Could you check a few things on this model? Use its own coordinates, in mm. Face numbers are marked on the shaded views. A direction names the side the tool comes from. Coordinates: 2 decimals unless noted, no trailing zeros. Write each loop counter-clockwise with the first axis right and the second up, starting at its lowest first coordinate (ties: lowest second). Pieces come first, ordered by that corner, then holes. Notation, with made-up numbers: M 5.5,26.25 L 29.5,26.25 A22 ccw 29.5,49.25 Z; hole C 58,89.25 d7. An arc over 180 degrees is marked long. Answer as CSV lines item,"result". Start each with the question number.
Item 1: We'd pull the mould along Z, two halves only. Please class the marked faces 3, 4, 5 and 6: +Z half, -Z half, draft (parallel to the pull), parting line (faces both ways), or undercut.
Item 2: On a 3-axis mill with a long thin cutter (end or side, diameter ignored), from which of +Z, -Z, +X, -X, +Y, -Y can I reach the whole of each face in a straight line? I mean the marked faces 1 and 2. Say none if no direction works.
Item 3: Suppose I cut it at B-B, the plane x = 6.5. Write out the boundary of the cut face in (y, z).
Item 4: If I drill on line 1 along X through (y, z) = (-12, 13.5); line 2 along Z through (x, y) = (15, -5.5); line 3 along Y through (x, z) = (1, 33), over which ranges is the centre line in solid material (lowest first)? Write a range as [from, to].
Item 5: I'm going to push a flat-ended pin straight in: P1, Ø10, axis at x = 25.5, z = -10, coming from the -Y side. Where does the tip first touch, or does it pass through?
Item 6: Suppose I cut it at C-C, the plane z = -44.5. Write out the boundary of the cut face in (x, y).
Item 7: Suppose I cut it at A-A, the plane y = -15.25. Write out the boundary of the cut face in (x, z), and give its area (3 significant figures).
```python
from build123d import *

# Parameters (mm, degrees)
F0_W     = 69.494404
F0_H     = 106.984802
F1_DEPTH = 25.4
F2_R     = 5.08
F3_T     = -2.54


with BuildPart() as f1:
    # F0 (on Front) → F1 (new body)
    with BuildSketch(Plane.XZ):
        Rectangle(F0_W, F0_H)
    extrude(amount=F1_DEPTH)

    # F2
    f2_edges = [f1.edges().sort_by_distance(p)[0] for p in [
        (-34.747202, -12.7, 53.492401),
        (-34.747202, -12.7, -53.492401),
        (34.747202, -12.7, 53.492401),
        (34.747202, -12.7, -53.492401),
    ]]
    fillet(f2_edges, radius=F2_R)

    # F3
    f3_openings = [f1.faces().sort_by_distance(p)[0] for p in [
        (0, -25.4, 0),
    ]]
    offset(amount=F3_T, openings=f3_openings)


solid = f1.part
```
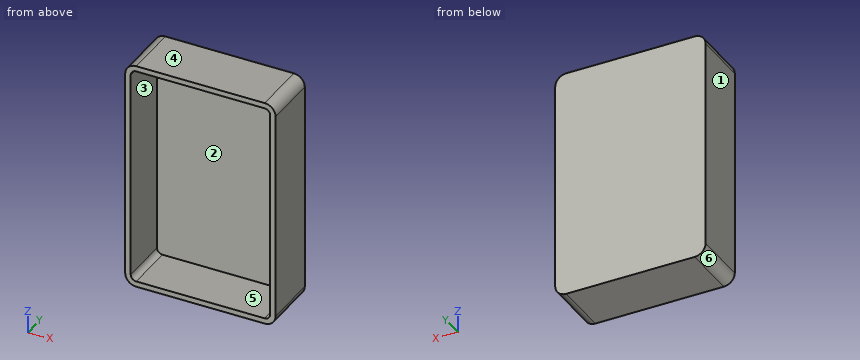
Ans:
1,face 3,"undercut"
1,face 4,"+Z half"
1,face 5,"undercut"
1,face 6,"-Z half"
2,face 1,"+Z, -Z, -X, +Y, -Y"
2,face 2,"-Y"
3,outline,"M -25.4,-53.49 L 0,-53.49 L 0,53.49 L -25.4,53.49 L -25.4,50.95 L -2.54,50.95 L -2.54,-50.95 L -25.4,-50.95 Z"
4,line 1,"x = [-34.75, -32.21], [32.21, 34.75]"
4,line 2,"z = [-53.49, -50.95], [50.95, 53.49]"
4,line 3,"y = [-2.54, 0]"
5,P1,"stops at y = -2.54"
6,outline,"M -34.75,-25.4 L -32.21,-25.4 L -32.21,-2.54 L 32.21,-2.54 L 32.21,-25.4 L 34.75,-25.4 L 34.75,0 L -34.75,0 Z"
7,outline,"M -34.75,-48.41 A5.08 ccw -29.67,-53.49 L 29.67,-53.49 A5.08 ccw 34.75,-48.41 L 34.75,48.41 A5.08 ccw 29.67,53.49 L -29.67,53.49 A5.08 ccw -34.75,48.41 Z; hole M -32.21,-48.41 A2.54 ccw -29.67,-50.95 L 29.67,-50.95 A2.54 ccw 32.21,-48.41 L 32.21,48.41 A2.54 ccw 29.67,50.95 L -29.67,50.95 A2.54 ccw -32.21,48.41 Z"
7,area,"854 mm^2"
